Autodesk Inventor part; units mm, degrees
ref_plane "YZ Plane" through (0, 0, 0) normal (1, 0, 0) x (0, 1, 0)
ref_plane "XZ Plane" through (0, 0, 0) normal (0, 1, 0) x (-1, 0, 0)
ref_plane "XY Plane" through (0, 0, 0) normal (0, 0, 1) x (1, 0, 0)
sketch "Sketch1" plane through (0, 0, 0) normal (0, 1, 0) x (-1, 0, 0)
  line L0 (381.5, 268.3) -> (-381.5, 268.3)
  line L1 (-381.5, 268.3) -> (-381.5, -268.3)
  line L2 (-381.5, -268.3) -> (381.5, -268.3)
  line L3 (381.5, -268.3) -> (381.5, 268.3)
  line L4 (381.5, 268.3) -> (-381.5, -268.3) construction
  line L5 (-381.5, 268.3) -> (381.5, -268.3) construction
  point P0 (0, 0)
  dimension "d0" = 763
  dimension "d1" = 536.6
extrude "Plate1" add sketch "Sketch1" along normal blind 0.9
sketch "Sketch2" plane through (381.5, 0, 267.4) normal (0, 0, 1) x (1, 0, 0)
  line L0 (-763, 0) -> (0, 0)
  line L1 (0, 0) -> (0, 20)
  line L2 (0, 20) -> (-763, 20)
  line L3 (-763, 20) -> (-763, 0)
edge flange "Flange1" height 20 angle 90 thickness 0.9 bend radius 1.008 thickness toward (0, 0, 1) relief tear relief width 0.9 relief depth 0.45 corner gap 1.008 corner form 0 edges at (0, 0.9, 268.3) (0, 0.9, -268.3) wall of the first edge with corners at (-381.5, 0, 267.4) (381.5, 0, 267.4) (381.5, 20, 267.4) (-381.5, 20, 267.4)
bend "Bend1"
corner "Corner1"
sketch "Sketch3" plane through (-381.5, 20, 268.3) normal (0, 0, 1) x (1, 0, 0)
  circle A0 centre (381.5, -11) radius 1.7
  circle A1 centre (61.5, -11) radius 1.7
  line L0 (0, 0) -> (763, 0)
  point P0 (381.5, -20)
  point P1 (701.5, -11)
  dimension "d20" = 11
  dimension "d41" = 320
  dimension "d42" = 320
hole "Hole1" at (-320, 9, 268.3) at (0, 9, 268.3) at (320, 9, 268.3) direction (0, 0, -1) diameter 6 end through all
sketch "Sketch6" plane through (0, 0, 0) normal (0, -1, 0) x (1, 0, 0)
  line L0 (381.5, -268.3) -> (-381.5, -268.3)
  line L1 (329.5, -203.3) -> (329.5, -268.3)
  line L2 (329.5, -268.3) -> (381.5, -268.3)
  line L3 (381.5, -268.3) -> (381.5, -203.3)
  line L4 (329.5, -203.3) -> (381.5, -203.3)
  point P0 (0, 0)
  dimension "d39" = 52
  dimension "d44" = 65
extrude "Cut1" cut sketch "Sketch6" against normal through all
fillet "Corner Round1" radius 2 6 edges at (329.5, 20, -267.85) (381.5, 20, 267.85) (-381.5, 20, -267.85) (-381.5, 20, 267.85) (329.5, 0.45, -203.3) (381.5, 0.45, -203.3)
sketch "Sketch8" plane through (0, 0, 0) normal (0, -1, 0) x (1, 0, 0)
  circle A0 centre (325.5, -199.3) radius 1.8
  circle A1 centre (374, -197.8) radius 1.8
  circle A2 centre (324, -260.5) radius 1.8
  arc A3 (377, -268) -> (381.5, -263.5) centre (377, -263.5) ccw
  line L0 (381.5, -263.5) -> (381.5, -193.3)
  arc A4 (381.5, -193.3) -> (378.5, -190.3) centre (378.5, -193.3) ccw
  line L1 (378.5, -190.3) -> (322.5, -190.3)
  arc A5 (322.5, -190.3) -> (316.5, -196.3) centre (322.5, -196.3) ccw
  line L2 (316.5, -196.3) -> (316.5, -265)
  arc A6 (316.5, -265) -> (319.5, -268) centre (319.5, -265) ccw
  line L3 (319.5, -268) -> (377, -268)
  line L4 (379.5, -208.3) -> (379.5, -263)
  arc A7 (376.5, -266) -> (379.5, -263) centre (376.5, -263) ccw
  line L5 (376.5, -266) -> (334.5, -266)
  arc A8 (331.5, -263) -> (334.5, -266) centre (334.5, -263) ccw
  line L6 (331.5, -263) -> (331.5, -208.3)
  arc A9 (334.5, -205.3) -> (331.5, -208.3) centre (334.5, -208.3) ccw
  line L7 (334.5, -205.3) -> (376.5, -205.3)
  arc A10 (379.5, -208.3) -> (376.5, -205.3) centre (376.5, -208.3) ccw
  point P0 (0, 0)
hole "Hole2" at (374, 0, -197.8) at (325.5, 0, -199.3) at (324, 0, -260.5) direction (0, 1, 0) diameter 3.4 depth 0.9 tip angle 118
equation "\"d18\" = Thickness"
equation "\"d50\" = Thickness"
equation "\"d2\" = Thickness"
equation "\"d3\" = BendReliefWidth"
equation "\"d4\" = BendReliefDepth"
equation "\"d5\" = MinimumRemnant"
equation "\"d6\" = TransitionRadius"
equation "\"d9\" = BendRadius"
equation "\"d10\" = CornerReliefSize"
equation "\"d11\" = GapSize"
equation "\"d12\" = JacobiRadiusSize"
equation "\"BendReliefWidth\" = Thickness"
equation "\"BendReliefDepth\" = 0.5 * Thickness"
equation "\"CornerReliefSize\" = 4 * Thickness"
equation "\"MinimumRemnant\" = 2 * Thickness"
equation "\"TransitionRadius\" = BendRadius"
equation "\"JacobiRadiusSize\" = BendRadius"
equation "\"GapSize\" = Thickness"
properties part number "SP41V1 Cubre Base" material "Steel, Carbon"
The model under review builds one solid part; all positions refer to its coordinate system, in mm. A direction names the side the tool comes from. Round coordinates to 2 decimals unless told otherwise and drop trailing zeros. Write each loop counter-clockwise with the first axis right and the second up, starting at its lowest first coordinate (ties: lowest second). Pieces come first, ordered by that corner, then holes. Notation, with made-up numbers: (46, 14.25) - (94, 14.25) arc R16 cw to (94, 22.25) - close; hole circle Ø2 at (73, 86.5). An arc over 180 degrees is marked (long way). Use one line per item in the form item = value.
Q1. Consider section C-C (z = -180). State the section outline as (x, y) points.
Answer key:
outline = (-381.5, 0) - (381.5, 0) - (381.5, 0.9) - (-381.5, 0.9) - close
Q2. Tool access review of faces 1 (the flat face through (329.5, 0.3, -236.7)), 2 (the flat face through (5, 11, 267.4)), 3 (the flat face through (-31, 11, -268.3)): name each direction out of +Z, -Z, +X, -X, +Y, -Y from which nothing blocks a thin tool from reaching the whole face with its end or side.
Answer key:
face_1 = -Z, +X, +Y, -Y
face_2 = +X, -X, +Y
face_3 = -Z, +X, -X, +Y, -Y
Q3. For line 1 (X direction, y = 9, z = 267.75); line 2 (X direction, y = 9, z = -268); line 3 (Z direction, x = 158, y = 6.5), list the stretches that pass through material, from the lowest coordinate up. Write a range as [from, to].
Answer key:
line_1 = [-381.5, -323], [-317, -3], [3, 317], [323, 381.5]
line_2 = [-381.5, -323], [-317, -3], [3, 317], [323, 329.5]
line_3 = [-268.3, -267.4], [267.4, 268.3]
Q4. Consider section A-A (y = 9). State how many separate pieces and enclosed holes the cut face has, and give its area (3 significant figures).
Answer key:
separate_pieces = 8
enclosed_holes = 0
area = 1,290 mm2
Q5. Draft analysis for pull direction Z (two halves, no side actions). For faces 4 (the flat face through (381.5, 0.4, 34.6)), 5 (the flat face through (5, 11, 268.3)), 6 (the flat face through (5, 0.9, 4)), state which applies: +Z half, -Z half, draft (parallel to the pull), parting line (faces both ways), or undercut.
Answer key:
face_4 = draft
face_5 = +Z half
face_6 = undercut
Q6. Insertion check: pin 1 Ø4.5 at (x, z) = (325.5, -199.3) entering from +Y. The pin has a flat end and moves straight along its axis. Give the tip position at first contact, or say it passes through.
Answer key:
pin_1 = 0.9
Q7. Consider section B-B (x = -60.5). State the section outline as (y, z) points, and give its area (3 significant figures).
Answer key:
outline = (0, -266.39) arc R1.91 ccw to (1.91, -268.3) - (20, -268.3) - (20, -267.4) - (1.91, -267.4) arc R1.01 cw to (0.9, -266.39) - (0.9, 266.39) arc R1.01 cw to (1.91, 267.4) - (20, 267.4) - (20, 268.3) - (1.91, 268.3) arc R1.91 ccw to (0, 266.39) - close
area = 516 mm2
